CAD build for the part. Positions are in the model's coordinates, mm. A direction names the side the tool comes from. Give positions to 0.01 mm unless a question says otherwise; leave off trailing zeros. Order: outer loops, then holes, each group sorted by start corner. A loop starts at its lowest first (then second) coordinate and runs counter-clockwise, first axis right, second up. Notation, with made-up numbers: M 84.5,75 L 118.5,75 A18 ccw 118.5,86 Z; hole C 84.5,38.25 d5. An arc over 180 degrees is marked long. Put each result on its own line as item: value. Start each with the question number.
1) Cut at A-A (y = -21). Write the cut outline in (x, z), and give its area (3 significant figures).
2) Pin check, flat tips, straight feed: pin 1 (5 mm diameter, centred on y = -41, z = -9.5, fed in from -X); pin 2 (4 mm diameter, centred on y = -24, z = -12, fed in from +X); pin 3 (7 mm diameter, centred on x = 0, z = -4.5, fed in from +Y). Stop position of each tip, or through.
3) Two-plate mould, pull along Z, no slides. Class faces 1 (the face through (-5.22, -34.06, -2.96)), 2 (the face through (28, -9, -7)), 3 (the face through (-7.36, -10.11, -23.37)), 4 (the face through (25.284, -5.219, -13.151)): released by +Z, released by -Z, zero draft, split by the parting line, or undercut.
4) Cut at B-B (y = -44). Write the cut outline in (x, z).
5) Drill centre lines: line 1 (Y direction, x = 18.5, z = -22.5); line 2 (Z direction, x = -3, y = -8); line 3 (Z direction, x = -1, y = -7). Where is each one in solid material? Low to high. Write a range as [from, to].
6) Tool access for faces 5 (the face through (-3.604, -14.451, -11.446)), 6 (the face through (-31.232, -8.24, 4.101)), 7 (the face through (10, -30, 10)), 8 (the face through (28, -3, -7)): list every direction of +Z, -Z, +X, -X, +Y, -Y with a clear straight run to the whole face (end or side of a thin tool).
```python
from build123d import *

# Parameters (mm, degrees)
CUT_EXTRUDE_1_DEPTH = 50
CUT_EXTRUDE_2_DEPTH = 8
CHAMFER_1_SIZE      = 2


with BuildPart() as part:
    # 草图1 → 旋转1 (revolve)
    with BuildSketch(Plane.XY, mode=Mode.PRIVATE) as revolve_1_sk:
        Polygon((24.5, -30), (24.5, -20), (12, -20), (12, -11), (7.5, -11), (7.5, -3), (0, -3), (0, -20), (0, -30), (0, -38), (10, -38), (10, -30), align=None)
        Polygon((31.5, 0), (24.5, 0), (24.5, -20), (24.5, -30), (28.5, -30), (28.5, -20), (28.5, -9), (31.5, -9), (31.5, -7.5), (28.5, -7.5), (28.5, -3), (31.5, -3), align=None)
        Polygon((28.5, -30), (24.5, -30), (24.5, -50), (31.5, -50), (31.5, -47), (28.5, -47), (28.5, -42.5), (31.5, -42.5), (31.5, -41), (28.5, -41), align=None)
    revolve(revolve_1_sk.sketch.rotate(Axis((0, 0, 0), (0, 1, 0)), 90), axis=Axis((0, 0, 0), (0, 1, 0)))

    # 草图2 → 切除-拉伸1 (cut)
    with BuildSketch(Plane(origin=(0, -3, 0), x_dir=(1, 0, 0), z_dir=(0, 1, 0))):
        with BuildLine():
            Line((5.7, 1.5), (3.708099244, 1.5))
            ThreePointArc((3.708099244, 1.5), (-4, 0), (3.708099244, -1.5))
            Line((3.708099244, -1.5), (5.7, -1.5))
            Line((5.7, -1.5), (5.7, 1.5))
        make_face()
    extrude(amount=-CUT_EXTRUDE_1_DEPTH, mode=Mode.SUBTRACT)

    # 草图3 → 切除-拉伸2 (cut)
    with BuildSketch(Plane.XZ.offset(38)):
        Polygon((6.92820323, 0), (3.464101615, 6), (-3.464101615, 6), (-6.92820323, 0), (-3.464101615, -6), (3.464101615, -6), align=None)
    extrude(amount=-CUT_EXTRUDE_2_DEPTH, mode=Mode.SUBTRACT)

    # 倒角1
    chamfer_1_edges = [part.edges().sort_by_distance(p)[0] for p in [
        (0, -11, 7.5),
        (0, -20, 12),
        (0, -20, 24.5),
        (0, 0, 24.5),
        (0, -50, 24.5),
        (0, -30, 24.5),
        (0, -30, 10),
    ]]
    chamfer(chamfer_1_edges, length=CHAMFER_1_SIZE)


solid = part.part
```
Solution:
1. outline: C 0,0 d57; hole M 3.71,-1.5 L 5.7,-1.5 L 5.7,1.5 L 3.71,1.5 A4 ccw long Z
1. area: 2,500 mm²
2. pin 1: x = -30.71
2. pin 2: x = 26.69
2. pin 3: y = -3
3. face 1: undercut
3. face 2: zero draft
3. face 3: undercut
3. face 4: split by the parting line
4. outline: C 0,0 d57; hole C 0,0 d49
5. line 1: [-50, -47], [-42.5, -41], [-9, -7.5], [-3, 0]
5. line 2: [-31.36, -24.32], [-6.87, -2.65], [2.65, 6.87], [24.32, 31.36]
5. line 3: [-28.48, -24.48], [-7.43, -3.87], [3.87, 7.43], [24.48, 28.48]
6. face 5: +Y
6. face 6: +Y, -Y
6. face 7: -Y
6. face 8: none
